The drawing under review shows one solid part. Ordinate dimensions are in mm from its lowest x, y, z. Give positions to 0.01 mm unless a question says otherwise; leave off trailing zeros. Write each loop counter-clockwise with the first axis right and the second up, starting at its lowest first coordinate (ties: lowest second). Pieces come first, ordered by that corner, then holes. Notation, with made-up numbers: M -36,-9 L 21,-9 A32 ccw 21,28 Z; hole C 36,-26.75 d3. An arc over 180 degrees is marked long. One line per item, written item: value. Start each with the question number.
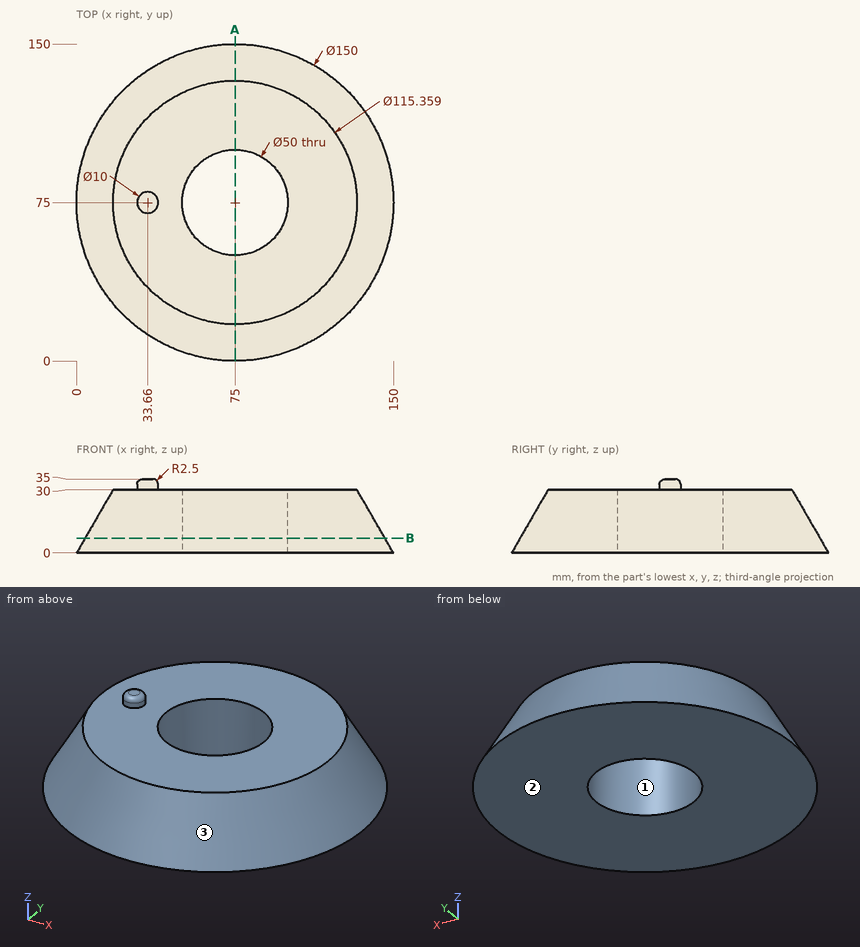
Q1. Wall thickness on line 1 (Y direction, x = 88, z = 16) (1 decimal); line 2 (Y direction, x = 75, z = 14); line 3 (Z direction, x = 48, y = 56): over which ranges is each line inside the solid? List them lowest first. Write a range as from..to.
Q2. For P1, Ø1.5, axis at x = 115.5, y = 75, coming from the +Z side; P2, Ø5, axis at x = 63.5, z = 13.5, coming from the +Y side; P3, Ø1, axis at x = 96, z = 11, coming from the +Y side, all flat-tipped, find the tip position at first contact; note any pin that passes through.
Q3. Take a section at B-B, the plane z = 7. Give the boundary of the cut face in (x, y), then the cut area to 3 significant figures.
Q4. Take a section at A-A, the plane x = 75. Give the boundary of the cut face in (y, z), then the cut area to 3 significant figures.
Q5. The part is to be moulded in two halves that separate along X. For the marked faces 1, 2 and 3, say which applies: pulls with the +X half, pulls with the -X half, needs draft (parallel to the pull), parting line crosses it, or undercut.
Results list:
1. line 1: y = 10.5..53.6, 96.4..139.5
1. line 2: y = 8.08..50, 100..141.92
1. line 3: z = 0..30
2. P1: stops at z = 30
2. P2: stops at y = 142.74
2. P3: stops at y = 140.7
3. outline: C 75,75 d141.92; hole C 75,75 d50
3. area: 13,900 mm^2
4. outline: M 0,0 L 50,0 L 50,30 L 17.32,30 Z; M 100,0 L 150,0 L 132.68,30 L 100,30 Z
4. area: 2,480 mm^2
5. face 1: undercut
5. face 2: needs draft
5. face 3: parting line crosses it
